Design review of the part shown in the three views and the two pictorial views. Dimensions are in mm from the part's minimum x, y and z. A direction names the side the tool comes from. Give positions to 0.01 mm unless a question says otherwise; leave off trailing zeros. Loops run counter-clockwise (first coordinate to the right, second up) from the corner with the lowest first, then second, coordinate; pieces in that order, holes last. Notation, with made-up numbers: (41.25, 68.25) -> (70.25, 68.25) arc R13 ccw to (70.25, 87.25) -> close; hole circle Ø9 at (63, 81). An arc over 180 degrees is marked (long way). Answer as CSV lines item,"result".
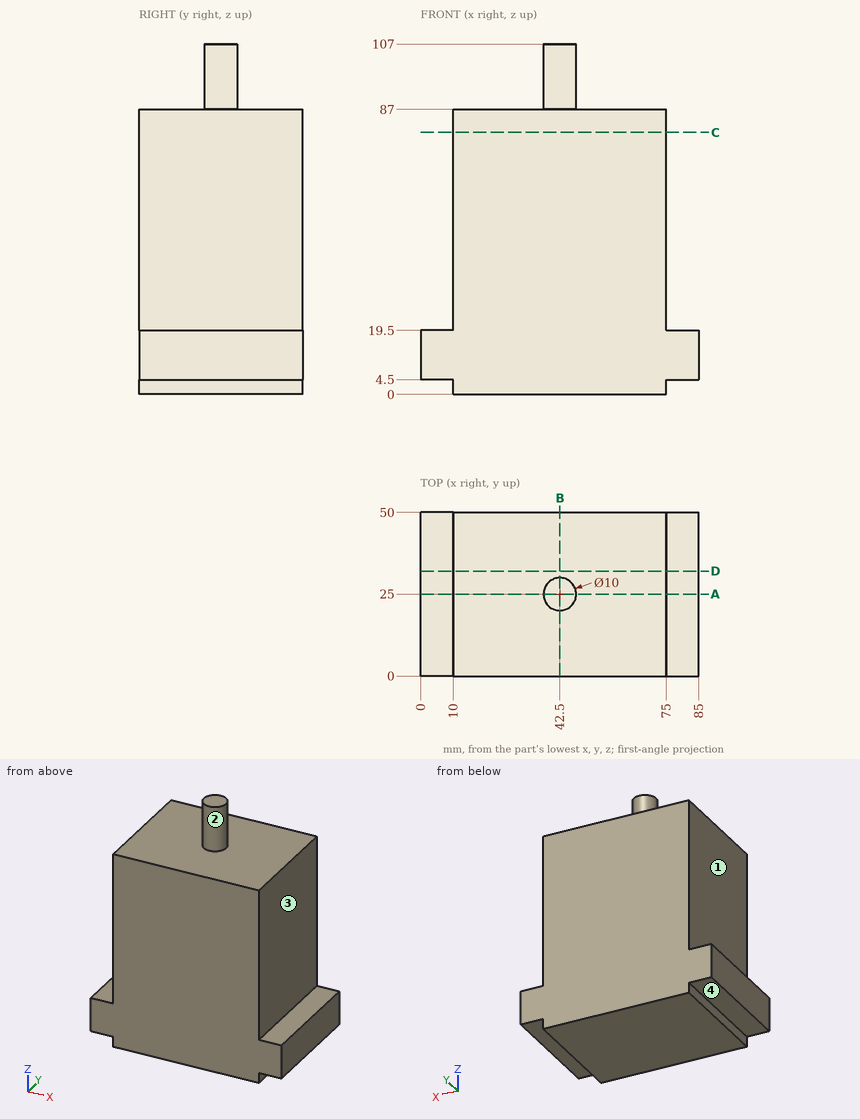
Q1. We need section C-C, the plane z = 80. State the section outline as (x, y) points.
Filled sheet:
outline,"(10, 0) -> (75, 0) -> (75, 50) -> (10, 50) -> close"
Q2. To check wall thickness, follow probe 1 along Z at (x, y) = (75.5, 7.5); probe 2 along X at (y, z) = (36, 46); probe 3 along Z at (x, y) = (68.5, 19). State the ranges of each line that lie inside material, in increasing order. Write a range as from..to.
Filled sheet:
probe 1,"z = 4.5..19.5"
probe 2,"x = 10..75"
probe 3,"z = 0..87"
Q3. For the marked faces 1, 2, 3 and 4, list the 3-axis set-ups (+Z, -Z, +X, -X, +Y, -Y) from which the entire face can be reached by the end or side of a thin tool; tool diameter is ignored.
Filled sheet:
face 1,"+Z, -X, +Y, -Y"
face 2,"+Z"
face 3,"+Z, +X, +Y, -Y"
face 4,"-Z, -X, +Y, -Y"
Q4. We need section D-D, the plane y = 32. State the section outline as (x, z) points, and give its area (4 significant figures).
Filled sheet:
outline,"(0, 4.5) -> (10, 4.5) -> (10, 0) -> (75, 0) -> (75, 4.5) -> (85, 4.5) -> (85, 19.5) -> (75, 19.5) -> (75, 87) -> (10, 87) -> (10, 19.5) -> (0, 19.5) -> close"
area,"5,955 mm^2"
Q5. Clearance check with flat-ended pins moving along their axes: pin 1 Ø1 at (y, z) = (19, 70.5) entering from +X; pin 2 Ø1 at (x, y) = (18, 19) entering from +Z; pin 3 Ø5 at (x, y) = (2.5, 15.5) entering from -Z. State where each tip first meets the part, or that it passes through.
Filled sheet:
pin 1,"stops at x = 75"
pin 2,"stops at z = 87"
pin 3,"stops at z = 4.5"
Q6. We need section A-A, the plane y = 25. State the section outline as (x, z) points, and give its area (4 significant figures).
Filled sheet:
outline,"(0, 4.5) -> (10, 4.5) -> (10, 0) -> (75, 0) -> (75, 4.5) -> (85, 4.5) -> (85, 19.5) -> (75, 19.5) -> (75, 87) -> (47.5, 87) -> (47.5, 107) -> (37.5, 107) -> (37.5, 87) -> (10, 87) -> (10, 19.5) -> (0, 19.5) -> close"
area,"6,155 mm^2"
Q7. We need section B-B, the plane x = 42.5. State the section outline as (y, z) points, and give its area (3 significant figures).
Filled sheet:
outline,"(0, 0) -> (50, 0) -> (50, 87) -> (30, 87) -> (30, 107) -> (20, 107) -> (20, 87) -> (0, 87) -> close"
area,"4,550 mm^2"
